For this review, take the finished solid that the model builds, in its own axes (mm). Face numbers are marked on the shaded views. A direction names the side the tool comes from. Give positions to 0.01 mm unless a question says otherwise; leave off trailing zeros. Loops run counter-clockwise (first coordinate to the right, second up) from the corner with the lowest first, then second, coordinate; pieces in that order, holes last.
Autodesk Inventor part; units mm, degrees
ref_plane "YZ Plane" through (0, 0, 0) normal (1, 0, 0) x (0, 1, 0)
ref_plane "XZ Plane" through (0, 0, 0) normal (0, 1, 0) x (-1, 0, 0)
ref_plane "XY Plane" through (0, 0, 0) normal (0, 0, 1) x (1, 0, 0)
sketch "草图1" plane through (0, 0, 0) normal (0, 0, 1) x (1, 0, 0)
  line L0 (-25.95, -15) -> (25.95, -15) construction
  line L1 (25.95, -15) -> (25.95, 15) construction
  line L2 (25.95, 15) -> (-25.95, 15) construction
  line L3 (-25.95, 15) -> (-25.95, -15) construction
  line L4 (-25.95, -15) -> (25.95, 15) construction
  line L5 (25.95, -15) -> (-25.95, 15) construction
  line L6 (0, 0) -> (-12.9865, 7.5067) construction
  line L7 (0, 0) -> (12.9865, 7.5067) construction
  line L8 (0, 0) -> (-12.9865, -7.5067) construction
  line L9 (0, 0) -> (12.9865, -7.5067) construction
  circle A0 centre (0, 0) radius 11.5
  line L10 (-20, -13.5) -> (20, -13.5)
  line L11 (20, -13.5) -> (20, 13.5)
  line L12 (20, 13.5) -> (-20, 13.5)
  line L13 (-20, 13.5) -> (-20, -13.5)
  line L14 (-20, -13.5) -> (20, 13.5) construction
  line L15 (20, -13.5) -> (-20, 13.5) construction
  circle A1 centre (12.9865, 7.5067) radius 2.5
  circle A2 centre (-12.9865, 7.5067) radius 2.5
  circle A3 centre (12.9865, -7.5067) radius 2.5
  dimension "d0" = 51.9
  dimension "d1" = 30
  dimension "d6" = 23
  dimension "d7" = 40
  dimension "d8" = 27
  dimension "d11" = 5
  dimension "d12" = 5
  dimension "d13" = 5
extrude "拉伸1" add sketch "草图1" along normal blind 4 contours L13 L12 L11 L10 | A1 | A2 | A3
hole "孔1" at (-12.9865, 7.5067, 0) at (12.9865, 7.5067, 0) at (12.9865, -7.5067, 0) at (-12.9865, -7.5067, 0) at (0, 0, 0) direction (0, 0, 1) diameter 4.94 depth 3
sketch "草图2" plane through (0, 0, 4) normal (0, 0, 1) x (1, 0, 0)
  point P0 (0, 0)
  point P1 (0, 0)
hole "孔2" at (0, 0, 4) direction (0, 0, -1) diameter 25.4 depth 1.1
sketch "草图3" plane through (0, 0, 4) normal (0, 0, 1) x (1, 0, 0)
  point P0 (0, 0)
equation "\"折弯半径\" = 厚度"
equation "\"折弯释压宽度\" = 厚度"
equation "\"折弯释压深度\" = 0.5 * 厚度"
equation "\"拐角释压尺寸\" = 4 * 厚度"
equation "\"最小余量\" = 2 * 厚度"
equation "\"过渡半径\" = 折弯半径"
equation "\"Jacobi半径尺寸\" = 折弯半径"
equation "\"间隙大小\" = 厚度"
properties part number "zhunzhiguan2"
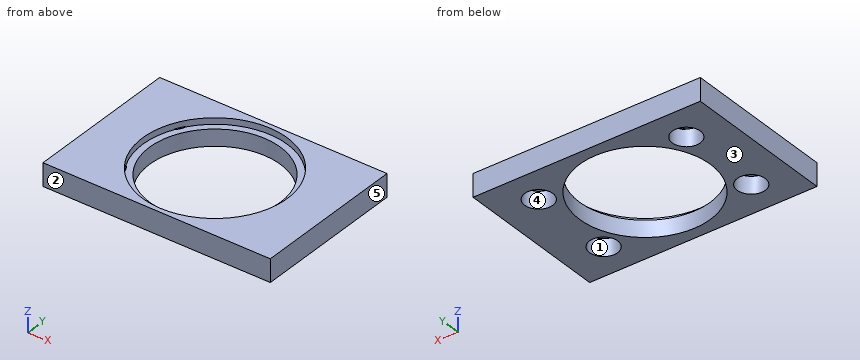
Q1. Consider section D-D on y = -8. Give the boundary of the cut face in (x, z), plus the area to 3 significant figures.
Answers:
outline: (-20, 0) - (-15.41, 0) - (-15.41, 3) - (-10.57, 3) - (-10.57, 0) - (-8.26, 0) - (-8.26, 2.9) - (-9.86, 2.9) - (-9.86, 4) - (-20, 4) - close; (8.26, 0) - (10.57, 0) - (10.57, 3) - (15.41, 3) - (15.41, 0) - (20, 0) - (20, 4) - (9.86, 4) - (9.86, 2.9) - (8.26, 2.9) - close
area: 61.3 mm2
Q2. For pin 1 Ø14 at (x, y) = (0, 0) entering from +Z; pin 2 Ø4 at (x, y) = (12.99, 7.51) entering from -Z; pin 3 Ø12.5 at (x, y) = (-1.5, 6) entering from +Z, all flat-tipped, find the tip position at first contact; note any pin that passes through.
Answers:
pin 1: passes through
pin 2: stops at z = 3
pin 3: stops at z = 2.9
Q3. Consider section B-B on y = 0. Give the boundary of the cut face in (x, z).
Answers:
outline: (-20, 0) - (-11.5, 0) - (-11.5, 2.9) - (-12.7, 2.9) - (-12.7, 4) - (-20, 4) - close; (11.5, 0) - (20, 0) - (20, 4) - (12.7, 4) - (12.7, 2.9) - (11.5, 2.9) - close
Q4. Consider section A-A on x = 0. Give the boundary of the cut face in (y, z).
Answers:
outline: (-13.5, 0) - (-11.5, 0) - (-11.5, 2.9) - (-12.7, 2.9) - (-12.7, 4) - (-13.5, 4) - close; (11.5, 0) - (13.5, 0) - (13.5, 4) - (12.7, 4) - (12.7, 2.9) - (11.5, 2.9) - close
Q5. Machinability: for the marked faces 1 and 2, which of the approach directions +Z, -Z, +X, -X, +Y, -Y give a long, thin tool a straight path to every point of the face, cutting with its end or side? Answer none if there is none.
Answers:
face 1: -Z
face 2: +Z, -Z, +X, -X, -Y
Q6. Consider section C-C on z = 1.4. Give the boundary of the cut face in (x, y), plus the area to 3 significant figures.
Answers:
outline: (-20, -13.5) - (20, -13.5) - (20, 13.5) - (-20, 13.5) - close; hole circle Ø4.94 at (-12.99, -7.51); hole circle Ø4.94 at (-12.99, 7.51); hole circle Ø23 at (0, 0); hole circle Ø4.94 at (12.99, -7.51); hole circle Ø4.94 at (12.99, 7.51)
area: 588 mm2
Q7. Mouldability with a two-part tool opening along X and no side actions: class the marked faces 3, 4 and 5 as +X half, -X half, draft (parallel to the pull), parting line (faces both ways), or undercut.
Answers:
face 3: draft
face 4: undercut
face 5: +X half
Q8. For probe 1 along X at (y, z) = (0, 3.6); probe 2 along Y at (x, z) = (0, 3.65); probe 3 along X at (y, z) = (7.5, 1.85), list the stretches that pass through material, from the lowest coordinate up.
Answers:
probe 1: x = -20 to -12.7, 12.7 to 20
probe 2: y = -13.5 to -12.7, 12.7 to 13.5
probe 3: x = -20 to -15.46, -10.52 to -8.72, 8.72 to 10.52, 15.46 to 20
